Check sheet for the modelled part. Datum: model origin and axes. Units: mm. A direction names the side the tool comes from. Give positions to 0.01 mm unless a question says otherwise; leave off trailing zeros. Loops run counter-clockwise (first coordinate to the right, second up) from the corner with the lowest first, then second, coordinate; pieces in that order, holes last. Notation, with made-up numbers: M 43,80 L 83,80 A18 cw 83,104 Z; hole C -20,4 d5. An arc over 180 degrees is marked long. Write each question's results on one line, items separated by ' | '. Start each with the question number.
1. Sectioned sample at C-C on y = 16. Record the cut outline in (x, z), and give its area (3 significant figures).
2. Draft check along Z on faces 3 (the flat face through (-2, 0, 1.5)), 4 (the flat face through (1, 0, -4.5)), 5 (the flat face through (1, 28, 0)). Enter one of: pulls with the +Z half, pulls with the -Z half, needs draft (parallel to the pull), parting line crosses it, or undercut.
3. Material ranges on line 1 along Y through (x, z) = (-29.5, -1); line 2 along Z through (x, y) = (22.5, -11.5); line 3 along X through (y, z) = (14, -1.25), recorded low to high.
4. Sectioned sample at D-D on z = 7.5. Record the cut outline in (x, y).
5. Sectioned sample at B-B on y = 0. Record the cut outline in (x, z).
6. Sectioned sample at A-A on x = 45. Record the cut outline in (y, z).
7. Tool access check on faces 1 (the flat face through (-2, -25, 0)), 2 (the flat face through (60, 0, 2)). Record the directions out of +Z, -Z, +X, -X, +Y, -Y that give a thin tool (end or side, any length) a straight path to the whole face; none if there is none.
8. Go/stop test with a flat-tipped pin: pin 1 (8 mm diameter, centred on x = 37, y = 11.5, fed in from +Z). Record where the tip stops, or that it passes through.
```python
from build123d import *

# Parameters (mm, degrees)
F1_DEPTH = 60
F2_W     = 50
F2_H     = 3
F3_DEPTH = 117


with BuildPart() as f1:
    # F0 (on Right) → F1 (new body, symmetric)
    with BuildSketch(Plane.YZ):
        with BuildLine():
            Line((-28, -4.5), (28, -4.5))
            Line((28, -4.5), (28, 4.5))
            ThreePointArc((28, 4.5), (0, 8.966381), (-28, 4.5))
            Line((-28, 4.5), (-28, -4.5))
        make_face()
    extrude(amount=F1_DEPTH, both=True)

    # F2 (on face) → F3 (cut)
    with BuildSketch(Plane(origin=(-60, 0, 0), x_dir=(0, -1, 0), z_dir=(-1, 0, 0))):
        Rectangle(F2_W, F2_H)
    extrude(amount=-F3_DEPTH, mode=Mode.SUBTRACT)


solid = f1.part
```
Output values:
1) outline: M -60,-4.5 L 60,-4.5 L 60,7.53 L -60,7.53 L -60,1.5 L 57,1.5 L 57,-1.5 L -60,-1.5 Z | area: 1,090 mm2
2) face 3: undercut | face 4: pulls with the -Z half | face 5: needs draft
3) line 1: -28 to -25, 25 to 28 | line 2: -4.5 to -1.5, 1.5 to 8.23 | line 3: 57 to 60
4) outline: M -60,-16.18 L 60,-16.18 L 60,16.18 L -60,16.18 Z
5) outline: M -60,-4.5 L 60,-4.5 L 60,8.97 L -60,8.97 L -60,1.5 L 57,1.5 L 57,-1.5 L -60,-1.5 Z
6) outline: M -28,-4.5 L 28,-4.5 L 28,4.5 A90 ccw -28,4.5 Z; hole M -25,-1.5 L 25,-1.5 L 25,1.5 L -25,1.5 Z
7) face 1: -X | face 2: +Z, -Z, +X, +Y, -Y
8) pin 1: z = 8.65
